Build history of the part. All positions in model axes, mm. A direction names the side the tool comes from. Give positions to 0.01 mm unless a question says otherwise; leave off trailing zeros. Write each loop counter-clockwise with the first axis right and the second up, starting at its lowest first coordinate (ties: lowest second). Pieces come first, ordered by that corner, then holes. Notation, with made-up numbers: M -33.5,39.5 L -24.5,39.5 A29 ccw -24.5,76.5 Z; hole C -12.75,0.25 d2. An arc over 180 degrees is marked long. Return JSON: item names as keys, results as strings. Group by question number.
Q1. Band-saw the part on B-B, the plane x = -4. Give the cut face in (y, z), then the cut area to 3 significant figures.
Q2. Band-saw the part on D-D, the plane y = -8.75. Give the cut face in (x, z), then the cut area to 3 significant figures.
Q3. Pull direction X, two halves, no side cores. Call faces 1 (the cylindrical face through (-30.5, -2, -29)), 2 (the cylindrical face through (-35.18, -1.97, -37.1)), 3 (the cylindrical face through (-7.58, -7.4, -5.81)), 4 (the flat face through (-10, 0, -10)): +X half, -X half, draft (parallel to the pull), parting line (faces both ways), or undercut.
Q4. Band-saw the part on A-A, the plane z = 6.5. Give the cut face in (x, y), then the cut area to 3 significant figures.
Q5. Band-saw the part on C-C, the plane y = -2. Give the cut face in (x, z), then the cut area to 3 significant figures.
Q6. Tool access for faces 5 (the cylindrical face through (12.932, -9.423, -5.362)), 6 (the flat face through (-3.31, -15, -9.14)): list every direction of +Z, -Z, +X, -X, +Y, -Y with a clear straight run to the whole face (end or side of a thin tool).
Q7. Flat gauge pins, fed straight in: pin 1 Ø3 at (x, y) = (-20.5, -2.5) entering from +Z; pin 2 Ø1 at (y, z) = (-4, 7) entering from +X; pin 3 Ø5 at (y, z) = (-4, -19) entering from -X. Where does each tip first touch, or does it go through?
Q8. Wall check: probe 1 along Z at (x, y) = (0, -9); probe 2 along Y at (x, z) = (-27, -20.5); probe 3 along Z at (x, y) = (-4.5, -4.75). Give the ranges that are in metal, low to high.
from build123d import *

# Parameters (mm, degrees)
F0_R     = 14
F0_R_2   = 9.55
F1_DEPTH = 15
F0_R_3   = 2.5
F2_DEPTH = 4


with BuildPart() as f1:
    # F0 (on Front) → F1 (new body)
    with BuildSketch(Plane.XZ):
        Circle(F0_R)
        Circle(F0_R_2, mode=Mode.SUBTRACT)
    extrude(amount=F1_DEPTH)

    # F0 (on Front) → F2 (join)
    with BuildSketch(Plane.XZ):
        with BuildLine():
            ThreePointArc((11.425317, -13.255645), (12.341197, 12.407451), (-13.316628, 11.354181))
            Line((-13.316628, 11.354181), (-36.645094, -27.632273))
            ThreePointArc((-36.645094, -27.632273), (-35.06435, -37.199789), (-25.367135, -37.210734))
            Line((-25.367135, -37.210734), (11.425317, -13.255645))
        make_face()
        with Locations((-30.209284, -31.483292)):
            Circle(F0_R_3, mode=Mode.SUBTRACT)
        Circle(F0_R, mode=Mode.SUBTRACT)
    extrude(amount=F2_DEPTH)


solid = f1.part
From the geometry:
{
 "1": {"outline": "M -15,-13.42 L -4,-13.42 L -4,-23.3 L 0,-23.3 L 0,-8.67 L -15,-8.67 Z; M -15,8.67 L 0,8.67 L 0,17.04 L -4,17.04 L -4,13.42 L -15,13.42 Z", "area": "196 mm^2"},
 "2": {"outline": "C 0,0 d28; hole C 0,0 d19.1", "area": "329 mm^2"},
 "3": {"face 1": "undercut", "face 2": "parting line", "face 3": "undercut", "face 4": "draft"},
 "4": {"outline": "M -16.22,-4 L -12.4,-4 L -12.4,-15 L -7,-15 L -7,0 L -16.22,0 Z; M 7,-15 L 12.4,-15 L 12.4,-4 L 16.25,-4 L 16.25,0 L 7,0 Z", "area": "193 mm^2"},
 "5": {"outline": "M -36.65,-27.63 A7.5 ccw -25.37,-37.21 L 11.43,-13.26 A17.5 ccw long -13.32,11.35 Z; hole C -30.21,-31.48 d5; hole C 0,0 d19.1", "area": "1,370 mm^2"},
 "6": {"face 5": "-Y", "face 6": "+Z, -Z, +X, -X, -Y"},
 "7": {"pin 1": "stops at z = 1.86", "pin 2": "stops at x = 16.25", "pin 3": "stops at x = -32.98"},
 "8": {"probe 1": "z = -14 to -9.55, 9.55 to 14", "probe 2": "y = -4 to 0", "probe 3": "z = -13.26 to -8.42, 8.42 to 13.26"}
}
